from build123d import *

# Parameters (mm, degrees)
NECK_SKETCH_R = 4.5
NECK_DEPTH    = 61
TOP_ROUND_R   = 8
BLEND_R       = 0.5


with BuildPart() as part:
    # Outside Profile_Sketch → Outside Profile (revolve)
    with BuildSketch(Plane.XY, mode=Mode.PRIVATE) as outside_profile_sk:
        Polygon((0, 0), (-18, 0), (-18, -55.9), (-4.5, -58.9), (0, -58.9), align=None)
    revolve(outside_profile_sk.sketch.rotate(Axis((0, 0, 0), (0, -1, 0)), 270), axis=Axis((0, 0, 0), (0, -1, 0)))

    # Neck_Sketch → Neck (add)
    with BuildSketch(Plane(origin=(0, 0, 0), x_dir=(1, 0, 0), z_dir=(0, 1, 0))):
        with Locations(Location((0, 0, 0), (0, 0, 270))):
            Circle(NECK_SKETCH_R)
    extrude(amount=-NECK_DEPTH)

    # Top Round
    top_round_edges = [part.edges().sort_by_distance(p)[0] for p in [
        (0, -55.9, -18),
    ]]
    fillet(top_round_edges, radius=TOP_ROUND_R)

    # Blend
    blend_edges = [part.edges().sort_by_distance(p)[0] for p in [
        (0, -58.9, -4.5),
    ]]
    fillet(blend_edges, radius=BLEND_R)

    # Shell_Sketch → Shell (revolve, cut)
    with BuildSketch(Plane.XY):
        with BuildLine():
            Line((-4.283069542, -57.92381294), (0, -57.92381294))
            Line((0, -57.92381294), (0, 0))
            Line((0, 0), (-17, 0))
            Line((-17, 0), (-17, -49.482627149))
            ThreePointArc((-17, -49.482627149), (-15.460292686, -53.862718904), (-11.518513205, -56.31593657))
            Line((-11.518513205, -56.31593657), (-4.283069542, -57.92381294))
        make_face()
    revolve(axis=Axis((0, 0, 0), (0, -1, 0)), mode=Mode.SUBTRACT)


solid = part.part
The model under review builds one solid part; all positions refer to its coordinate system, in mm. A direction names the side the tool comes from. Round coordinates to 2 decimals unless told otherwise and drop trailing zeros. Write each loop counter-clockwise with the first axis right and the second up, starting at its lowest first coordinate (ties: lowest second). Pieces come first, ordered by that corner, then holes. Notation, with made-up numbers: M -8,66.25 L 36,66.25 A14 cw 36,79.25 Z; hole C 24.5,1 d10. An arc over 180 degrees is marked long. Answer as CSV lines item,"result". Start each with the question number.
Q1. Tool access review of faces 1 (the face through (0, -57.924, 0)), 2 (the face through (1.352, -60.139, 4.292)), 3 (the face through (-7, 0, 16)): name each direction out of +Z, -Z, +X, -X, +Y, -Y from which nothing blocks a thin tool from reaching the whole face with its end or side.
Q2. Clearance check with flat-ended pins moving along their axes: P1, Ø5, axis at x = -7.5, z = 8.5, coming from the +Y side; P2, Ø3, axis at x = -11, z = 7.5, coming from the +Y side; P3, Ø3, axis at y = -41, z = 13.5, coming from the -X side. State where each tip first meets the part, or that it passes through.
Q3. Consider section A-A, the plane y = -25.5. Give the boundary of the cut face in (x, z).
Q4. Wall thickness on line 1 along X through (y, z) = (-28.5, 0); line 2 along X through (y, z) = (-33.5, -10.5); line 3 along Z through (x, y) = (3, -34): over which ranges is each line inside the solid? List them lowest first.
Result set:
1,face 1,"+Y"
1,face 2,"-Y"
1,face 3,"+Z, -Z, +X, -X, +Y"
2,P1,"stops at y = -55.34"
2,P2,"stops at y = -54.56"
2,P3,"stops at x = -13.42"
3,outline,"C 0,0 d36; hole C 0,0 d34"
4,line 1,"x = -18 to -17, 17 to 18"
4,line 2,"x = -14.62 to -13.37, 13.37 to 14.62"
4,line 3,"z = -17.75 to -16.73, 16.73 to 17.75"
